```python
from build123d import *

# Parameters (mm, degrees)
SKETCH1_R                       = 14.2875
BOSS_EXTRUDE1_DEPTH             = 4.7625
F_8_32_TAPPED_HOLE1_D           = 3.4544
F_8_32_TAPPED_HOLE1_DEPTH       = 19.05
F_8_32_TAPPED_HOLE1_CBORE_D     = 4.1656
F_8_32_TAPPED_HOLE1_CBORE_DEPTH = 15.875
F_8_32_TAPPED_HOLE1_TIP         = 1.037806461
F_8_32_TAPPED_HOLE2_D           = 3.4544
F_8_32_TAPPED_HOLE2_DEPTH       = 12.2936
F_8_32_TAPPED_HOLE2_TIP         = 1.037806461
CUT_EXTRUDE2_DEPTH              = 114.820982358
F_8_32_TAPPED_HOLE3_D           = 3.4544
F_8_32_TAPPED_HOLE3_DEPTH       = 12.2936
F_8_32_TAPPED_HOLE3_TIP         = 1.037806461
F_10_CLEARANCE_HOLE1_D          = 5.1054
F_10_CLEARANCE_HOLE1_DEPTH      = 9.525
F_10_CLEARANCE_HOLE1_TIP        = 1.533816902


with BuildPart() as part:
    # Sketch1 → Boss-Extrude1 (new, symmetric)
    with BuildSketch(Plane.XY):
        with BuildLine():
            Line((-44.45, 35.584432116), (-44.45, 0))
            Line((-44.45, 0), (44.45, 0))
            Line((44.45, 0), (44.45, 68.58))
            ThreePointArc((44.45, 68.58), (37.010512242, 86.540512242), (19.05, 93.98))
            Line((19.05, 93.98), (-38.1, 93.98))
            ThreePointArc((-38.1, 93.98), (-62.634515988, 75.154003746), (-50.8, 46.582954744))
            ThreePointArc((-50.8, 46.582954744), (-46.151477372, 41.934432116), (-44.45, 35.584432116))
        make_face()
        with Locations(Location((0, 68.58, 0), (0, 0, 180))):
            Circle(SKETCH1_R, mode=Mode.SUBTRACT)
        with Locations(Location((-38.1, 68.58, 0), (0, 0, 180))):
            Circle(SKETCH1_R, mode=Mode.SUBTRACT)
    extrude(amount=BOSS_EXTRUDE1_DEPTH, both=True)

    # #8-32 Tapped Hole1
    with Locations(Plane.XZ):
        with Locations((-19.05, 0), (19.05, 0)):
            CounterBoreHole(F_8_32_TAPPED_HOLE1_D / 2, F_8_32_TAPPED_HOLE1_CBORE_D / 2, F_8_32_TAPPED_HOLE1_CBORE_DEPTH, depth=F_8_32_TAPPED_HOLE1_DEPTH)
            with Locations((0, 0, -(F_8_32_TAPPED_HOLE1_DEPTH + F_8_32_TAPPED_HOLE1_TIP / 2))):  # 118° drill point
                Cone(0, F_8_32_TAPPED_HOLE1_D / 2, F_8_32_TAPPED_HOLE1_TIP, mode=Mode.SUBTRACT)

    # #8-32 Tapped Hole2
    with Locations(Plane(origin=(-44.45, 3.933791499, -1.696886329), x_dir=(0, 0, 1), z_dir=(-1, 0, 0))):
        with Locations((1.696886329, 15.116208501), (1.696886329, 2.416208501)):
            Hole(F_8_32_TAPPED_HOLE2_D / 2, depth=F_8_32_TAPPED_HOLE2_DEPTH)
            with Locations((0, 0, -(F_8_32_TAPPED_HOLE2_DEPTH + F_8_32_TAPPED_HOLE2_TIP / 2))):  # 118° drill point
                Cone(0, F_8_32_TAPPED_HOLE2_D / 2, F_8_32_TAPPED_HOLE2_TIP, mode=Mode.SUBTRACT)

    # Sketch7 → Cut-Extrude2 (cut, through all)
    with BuildSketch(Plane.XY.offset(4.7625)):
        with BuildLine():
            Line((-22.225, 44.45), (22.225, 44.45))
            ThreePointArc((22.225, 44.45), (26.715128061, 42.590128061), (28.575, 38.1))
            Line((28.575, 38.1), (28.575, 15.875))
            ThreePointArc((28.575, 15.875), (26.715128061, 11.384871939), (22.225, 9.525))
            Line((22.225, 9.525), (-22.225, 9.525))
            ThreePointArc((-22.225, 9.525), (-26.715128061, 11.384871939), (-28.575, 15.875))
            Line((-28.575, 15.875), (-28.575, 38.1))
            ThreePointArc((-28.575, 38.1), (-26.715128061, 42.590128061), (-22.225, 44.45))
        make_face()
    extrude(amount=-CUT_EXTRUDE2_DEPTH, mode=Mode.SUBTRACT)

    # #8-32 Tapped Hole3
    with Locations(Plane(origin=(44.45, 0, 0), x_dir=(0, 0, -1), z_dir=(1, 0, 0))):
        with Locations((0, 6.35), (0, 57.15)):
            Hole(F_8_32_TAPPED_HOLE3_D / 2, depth=F_8_32_TAPPED_HOLE3_DEPTH)
            with Locations((0, 0, -(F_8_32_TAPPED_HOLE3_DEPTH + F_8_32_TAPPED_HOLE3_TIP / 2))):  # 118° drill point
                Cone(0, F_8_32_TAPPED_HOLE3_D / 2, F_8_32_TAPPED_HOLE3_TIP, mode=Mode.SUBTRACT)

    # #10 Clearance Hole1
    with Locations(Plane(origin=(0, 0, -4.7625), x_dir=(-1, 0, 0), z_dir=(0, 0, -1))):
        with Locations((-25.4, 85.725), (25.4, 85.725), (38.1, 25.4), (-38.1, 25.4)):
            Hole(F_10_CLEARANCE_HOLE1_D / 2, depth=F_10_CLEARANCE_HOLE1_DEPTH)
            with Locations((0, 0, -(F_10_CLEARANCE_HOLE1_DEPTH + F_10_CLEARANCE_HOLE1_TIP / 2))):  # 118° drill point
                Cone(0, F_10_CLEARANCE_HOLE1_D / 2, F_10_CLEARANCE_HOLE1_TIP, mode=Mode.SUBTRACT)


solid = part.part
```
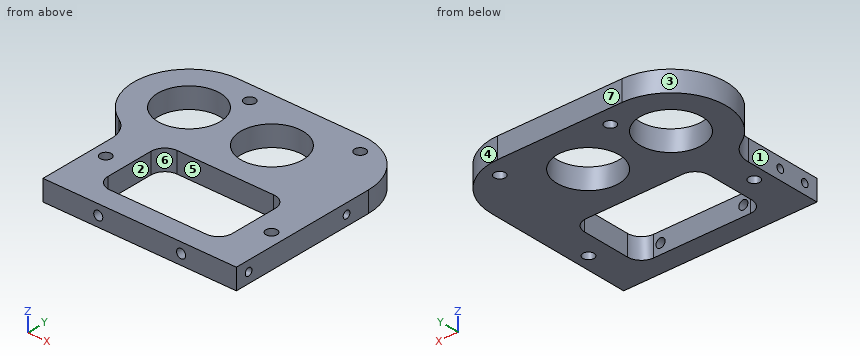
Model file for the job. Use its own axes, mm. Face numbers are marked on the shaded views. A direction names the side the tool comes from. Round coordinates to 2 decimals unless told otherwise and drop trailing zeros. Write each loop counter-clockwise with the first axis right and the second up, starting at its lowest first coordinate (ties: lowest second). Pieces come first, ordered by that corner, then holes. Notation, with made-up numbers: (-5, -21) -> (22, -21) arc R28 ccw to (22, 7) -> close; hole circle Ø11 at (5.25, -19). An arc over 180 degrees is marked (long way). Answer as CSV lines item,"result".
1. Slice it at A-A, the plane x = -19.05. State how many separate pieces and enclosed holes the cut face has, plus the area to 3 significant figures.
Resolved:
separate pieces,"3"
enclosed holes,"0"
area,"523 mm²"
2. Pin check, flat tips, straight feed: pin 1 Ø2 at (y, z) = (67, -3) entering from -X; pin 2 Ø4 at (y, z) = (6.35, 0) entering from +X; pin 3 Ø3 at (y, z) = (72, 0.5) entering from +X; pin 4 Ø5.5 at (y, z) = (57.15, 0) entering from -X. Stop position of each tip, or through.
Resolved:
pin 1,"x = -63.49"
pin 2,"x = 44.45"
pin 3,"x = 44.38"
pin 4,"x = -61.97"
3. Drill centre lines: line 1 (Y direction, x = -38.1, z = -2.5); line 2 (Y direction, x = 17, z = 2.25) (3 decimals); line 3 (Y direction, x = -0.5, z = 3) (3 decimals). Where is each one in solid material? Low to high.
Resolved:
line 1,"0 to 22.85, 27.95 to 54.29, 82.87 to 93.98"
line 2,"0 to 9.525, 44.45 to 93.98"
line 3,"0 to 9.525, 44.45 to 54.301, 82.859 to 93.98"
4. Mould opens along X. For the marked faces 4, 5, 6 and 7 say: +X half, -X half, draft (parallel to the pull), parting line (faces both ways), or undercut.
Resolved:
face 4,"+X half"
face 5,"undercut"
face 6,"undercut"
face 7,"draft"
5. Slice it at D-D, the plane x = 24. List the corners of the cut face in (y, z).
Resolved:
outline,"(0, -4.76) -> (9.78, -4.76) -> (9.78, 4.76) -> (0, 4.76) -> close; (44.2, -4.76) -> (83.59, -4.76) -> (83.59, 4.76) -> (44.2, 4.76) -> close; (87.86, -4.76) -> (93.49, -4.76) -> (93.49, 4.76) -> (87.86, 4.76) -> close"
6. Slice it at C-C, the plane x = -46.5. List the corners of the cut face in (y, z).
Resolved:
outline,"(42.5, -4.76) -> (57.02, -4.76) -> (57.02, 4.76) -> (42.5, 4.76) -> close; (80.14, -4.76) -> (92.55, -4.76) -> (92.55, 4.76) -> (80.14, 4.76) -> close"
7. Tool access for the marked faces 1, 2 and 3: list every direction of +Z, -Z, +X, -X, +Y, -Y with a clear straight run to the whole face (end or side of a thin tool).
Resolved:
face 1,"+Z, -Z, -X, -Y"
face 2,"+Z, -Z"
face 3,"+Z, -Z, -X"
